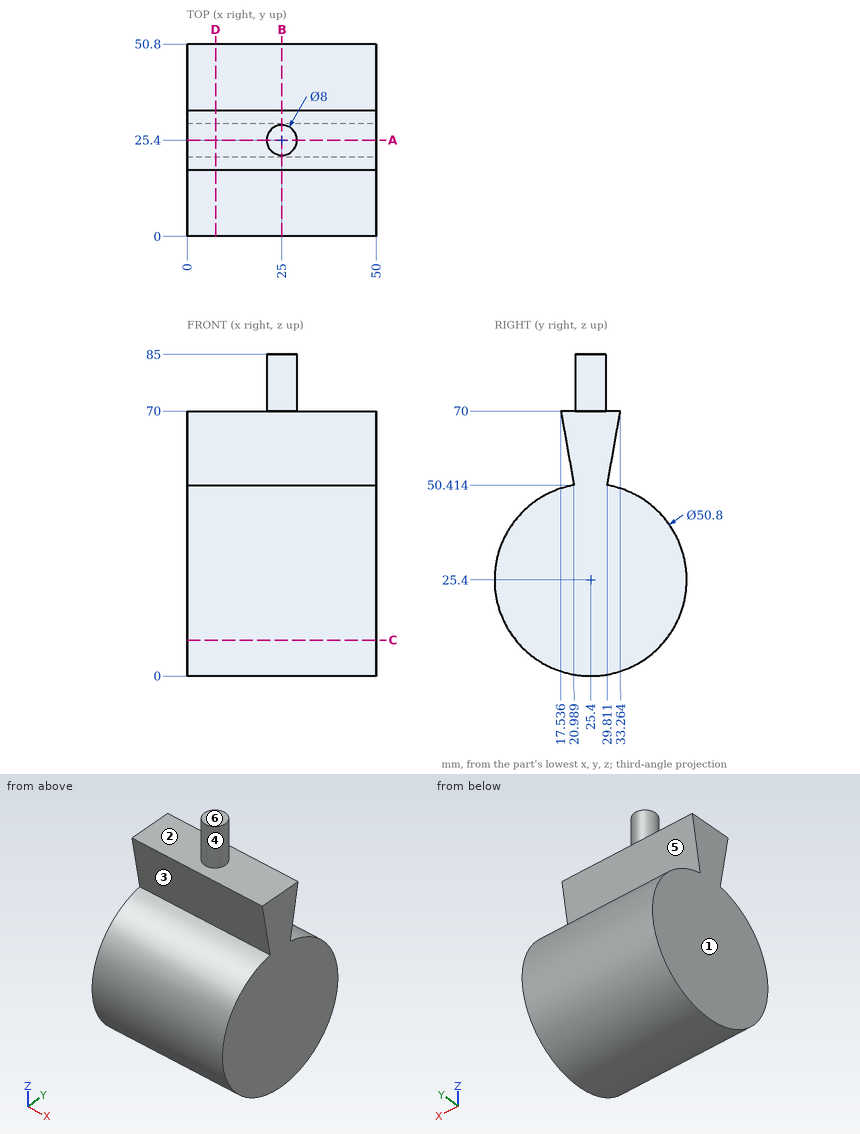
Geometry: see drawing. Coordinates: mm, zero at the bounding-box minimum. A direction names the side the tool comes from. Give positions to 0.01 mm unless a question says otherwise; leave off trailing zeros. Loops run counter-clockwise (first coordinate to the right, second up) from the corner with the lowest first, then second, coordinate; pieces in that order, holes last. Notation, with made-up numbers: (64, 77) -> (87, 77) arc R21 cw to (87, 91) -> close; hole circle Ø5 at (45.5, 71). An arc over 180 degrees is marked (long way). Put each result on its own line as item: value.
1. Cut plane C-C (z = 9.5). Return the cut outline in (x, y).
Taken from the geometry:
outline: (0, 5.59) -> (50, 5.59) -> (50, 45.21) -> (0, 45.21) -> close
2. Cut plane D-D (x = 7.5). Return the cut outline in (y, z), plus the area to 4 significant figures.
Taken from the geometry:
outline: (17.54, 70) -> (20.99, 50.41) arc R25.4 ccw (long way) to (29.81, 50.41) -> (33.26, 70) -> close
area: 2,265 mm2
3. Cut plane A-A (y = 25.4). Return the cut outline in (x, z), plus the area to 3 significant figures.
Taken from the geometry:
outline: (0, 0) -> (50, 0) -> (50, 70) -> (29, 70) -> (29, 85) -> (21, 85) -> (21, 70) -> (0, 70) -> close
area: 3,620 mm2
4. Set-up query: the marked faces 4, 5 and 6. Return all of +Z, -Z, +X, -X, +Y, -Y with unobstructed straight access to the full face (end or side cutting, diameter ignored); none if empty.
Taken from the geometry:
face 4: +Z
face 5: +X, -X, +Y
face 6: +Z, +X, -X, +Y, -Y
5. Pin query (flat end, axial travel): P1, Ø10, axis at y = 11, z = 73.5, coming from the +X side; P2, Ø1.5, axis at x = 29, z = 60, coming from the -Y side; P3, Ø3, axis at x = 36, y = 45, coming from the -Z side; P4, Ø8, axis at x = 17.5, y = 16.5, coming from the +Z side. Return the tip coordinate at first contact, or that it passes through.
Taken from the geometry:
P1: passes through
P2: stops at y = 19.17
P3: stops at z = 7.58
P4: stops at z = 70
6. Ray query, line 1 along Y through (x, z) = (33.5, 35.5) (1 decimal); line 2 along Y through (x, z) = (27, 4); line 3 along Z through (x, y) = (4.5, 11) (1 decimal). Return the intervals inside material, ascending. Write a range as [from, to].
Taken from the geometry:
line 1: y = [2.1, 48.7]
line 2: y = [11.72, 39.08]
line 3: z = [4.5, 46.3]
7. Cut plane B-B (x = 25). Return the cut outline in (y, z).
Taken from the geometry:
outline: (17.54, 70) -> (20.99, 50.41) arc R25.4 ccw (long way) to (29.81, 50.41) -> (33.26, 70) -> (29.4, 70) -> (29.4, 85) -> (21.4, 85) -> (21.4, 70) -> close
8. Pull-direction query (Z, two-part tool) for the marked faces 1, 2 and 3; classes: released by +Z, released by -Z, zero draft, split by the parting line, or undercut.
Taken from the geometry:
face 1: zero draft
face 2: released by +Z
face 3: undercut
